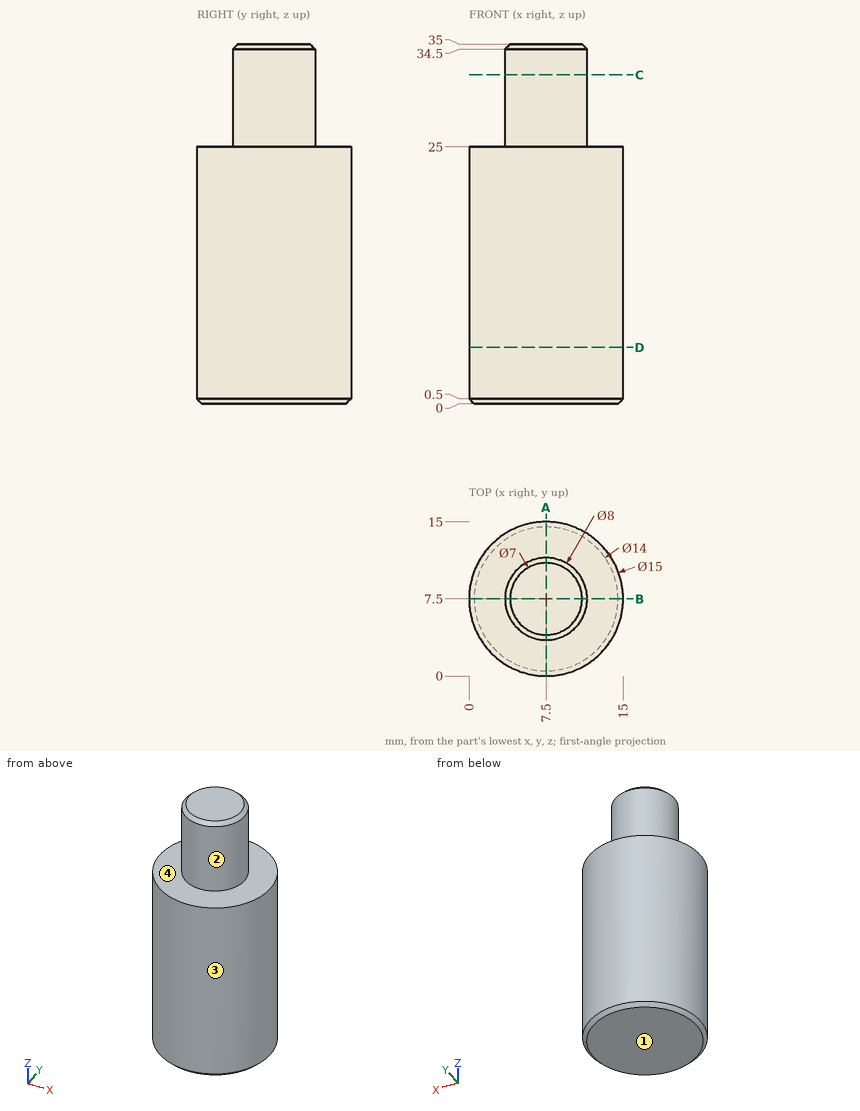
The drawing under review shows one solid part. Ordinate dimensions are in mm from its lowest x, y, z. A direction names the side the tool comes from. Round coordinates to 2 decimals unless told otherwise and drop trailing zeros. Loops run counter-clockwise (first coordinate to the right, second up) from the corner with the lowest first, then second, coordinate; pieces in that order, holes last. Notation, with made-up numbers: M 56,33.5 L 85,33.5 A13 cw 85,52.5 Z; hole C 69.25,-28.75 d3. An arc over 180 degrees is marked long. Answer as CSV lines item,"result". Start each with the question number.
Item 1: Mouldability with a two-part tool opening along X and no side actions: class the marked faces 1 and 2 as released by +X, released by -X, zero draft, split by the parting line, or undercut.
Item 2: Insertion check: P1, Ø3, axis at y = 5, z = 23.5, coming from the +X side; P2, Ø1, axis at y = 5.5, z = 26, coming from the -X side; P3, Ø1.5, axis at x = 4, y = 3, coming from the +Z side; P4, Ø7.5, axis at x = 5.5, y = 11, coming from the +Z side. Each pin has a flat end and moves straight along its axis. Give the tip position at first contact, or say it passes through.
Item 3: Consider section D-D (z = 5.5). Write out the cut boundary in (x, y), then the cut area to 3 significant figures.
Item 4: Consider section C-C (z = 32). Write out the cut boundary in (x, y).
Item 5: Wall thickness on line 1 (Z direction, x = 1.25, y = 9.5); line 2 (Z direction, x = 2, y = 2.75); line 3 (Y direction, x = 13.5, z = 10.5): over which ranges is each line inside the solid? List them lowest first. Write a range as [from, to].
Item 6: Consider section A-A (x = 7.5). Write out the cut boundary in (y, z), then the cut area to 4 significant figures.
Item 7: For the marked faces 3 and 4, list the 3-axis set-ups (+Z, -Z, +X, -X, +Y, -Y) from which the entire face can be reached by the end or side of a thin tool; tool diameter is ignored.
Answer:
1,face 1,"zero draft"
1,face 2,"split by the parting line"
2,P1,"stops at x = 14.93"
2,P2,"stops at x = 3.79"
2,P3,"stops at z = 25"
2,P4,"stops at z = 35"
3,outline,"C 7.5,7.5 d15"
3,area,"177 mm^2"
4,outline,"C 7.5,7.5 d8"
5,line 1,"z = [0, 25]"
5,line 2,"z = [0.27, 25]"
5,line 3,"y = [3, 12]"
6,outline,"M 0,0.5 L 0.5,0 L 14.5,0 L 15,0.5 L 15,25 L 11.5,25 L 11.5,34.5 L 11,35 L 4,35 L 3.5,34.5 L 3.5,25 L 0,25 Z"
6,area,"454.5 mm^2"
7,face 3,"+Z, -Z"
7,face 4,"+Z"
